```python
from build123d import *

# Parameters (mm, degrees)
BOSS_EXTRUDE1_DEPTH = 12
CUT_EXTRUDE1_DEPTH  = 7


with BuildPart() as part:
    # Sketch1 → Boss-Extrude1 (new body)
    with BuildSketch(Plane(origin=(0, 0, 0), x_dir=(1, 0, 0), z_dir=(0, 1, 0))):
        with BuildLine():
            Line((-420, 0), (-264.641016151, 0))
            ThreePointArc((-264.641016151, 0), (-255.980762114, 5), (-255.980762114, 15))
            ThreePointArc((-255.980762114, 15), (-255.980762114, 25), (-247.320508076, 30))
            Line((-247.320508076, 30), (-207.320508076, 30))
            ThreePointArc((-207.320508076, 30), (-198.660254038, 25), (-198.660254038, 15))
            ThreePointArc((-198.660254038, 15), (-198.660254038, 5), (-190, 0))
            Line((-190, 0), (-140, 0))
            ThreePointArc((-140, 0), (1.07e-06, 140), (140, -2.139e-06))
            Line((140, -2.139e-06), (190, -2.149e-06))
            ThreePointArc((190, -2.149e-06), (198.660254037, -5.000002151), (198.660254035, -15.000002151))
            ThreePointArc((198.660254035, -15.000002151), (198.660254033, -25.000002151), (207.32050807, -30.000002153))
            Line((207.32050807, -30.000002153), (247.32050807, -30.000002161))
            ThreePointArc((247.32050807, -30.000002161), (255.980762108, -25.000002163), (255.98076211, -15.000002163))
            ThreePointArc((255.98076211, -15.000002163), (255.980762113, -5.000002163), (264.641016151, -2.165e-06))
            Line((264.641016151, -2.165e-06), (420, -2.196e-06))
            ThreePointArc((420, -2.196e-06), (1.098e-06, 420), (-420, 0))
        make_face()
    extrude(amount=BOSS_EXTRUDE1_DEPTH)

    # Sketch2 → Cut-Extrude1 (cut)
    with BuildSketch(Plane.XZ):
        with BuildLine():
            ThreePointArc((0, -140), (-3.501094948, -139.956215775), (-7, -139.824890488))
            Line((-7, -139.824890488), (-7, -419.941662615))
            ThreePointArc((-7, -419.941662615), (-3.500121543, -419.985415401), (0, -420))
            Line((0, -420), (0, -140))
        make_face()
    extrude(amount=-CUT_EXTRUDE1_DEPTH, mode=Mode.SUBTRACT)


solid = part.part
```
Build history of the part. All positions in model axes, mm. Round coordinates to 2 decimals unless told otherwise and drop trailing zeros. Write each loop counter-clockwise with the first axis right and the second up, starting at its lowest first coordinate (ties: lowest second). Pieces come first, ordered by that corner, then holes.
1) Band-saw the part on A-A, the plane y = 9.5. List the corners of the cut face in (x, z).
2) Band-saw the part on D-D, the plane x = 313.5. List the corners of the cut face in (y, z).
3) Drill centre lines: probe 1 along X at (y, z) = (2.75, -164); probe 2 along X at (y, z) = (4.75, -333); probe 3 along Z at (x, y) = (-28, 5). Where is each one in solid material? Low to high.
4) Mould opens along X. For faces 1 (the flat face through (207, 0, -198)), 2 (the cylindrical face through (-3.079, 7.249, -139.966)), 3 (the cylindrical face through (9.2, 5.9, -419.9)) say: +X half, -X half, draft (parallel to the pull), parting line (faces both ways), or undercut.
5) Band-saw the part on C-C, the plane x = -122. List the corners of the cut face in (y, z).
6) Band-saw the part on B-B, the plane z = -197. List the corners of the cut face in (x, y).
7) Pin check, flat tips, straight feed: pin 1 (3.5 mm diameter, centred on x = -227, y = 6.5, fed in from +Z); pin 2 (3.5 mm diameter, centred on x = 175, y = 5, fed in from +Z); pin 3 (5.5 mm diameter, centred on y = 4, z = -219, fed in from -X). Stop position of each tip, or through.
Ans:
1. outline: (-420, 0) arc R420 ccw to (420, 0) - (264.64, 0) arc R10 cw to (255.98, 15) arc R10 ccw to (247.32, 30) - (207.32, 30) arc R10 ccw to (198.66, 15) arc R10 cw to (190, 0) - (140, 0) arc R140 cw to (-140, 0) - (-190, 0) arc R10 ccw to (-198.66, -15) arc R10 cw to (-207.32, -30) - (-247.32, -30) arc R10 cw to (-255.98, -15) arc R10 ccw to (-264.64, 0) - close
2. outline: (0, -279.5) - (12, -279.5) - (12, 0) - (0, 0) - close
3. probe 1: x = -386.66 to -7, 0 to 386.66
3. probe 2: x = -255.95 to -7, 0 to 255.95
3. probe 3: z = -419.07 to -137.17
4. face 1: draft
4. face 2: undercut
4. face 3: parting line
5. outline: (0, -401.89) - (12, -401.89) - (12, -68.67) - (0, -68.67) - close
6. outline: (-370.93, 0) - (-7, 0) - (-7, 7) - (0, 7) - (0, 0) - (370.93, 0) - (370.93, 12) - (-370.93, 12) - close
7. pin 1: stops at z = -30
7. pin 2: stops at z = 0
7. pin 3: stops at x = -360.05
